from build123d import *

# Parameters (mm, degrees)
F1_DEPTH = 30
F2_R     = 2
F3_R     = 2
F4_R     = 25
F5_DEPTH = 30
F6_W     = 50
F6_H     = 19.9247
F7_DEPTH = 60


with BuildPart() as f1:
    # F0 (on Front) → F1 (new body, symmetric)
    with BuildSketch(Plane.XZ):
        with BuildLine():
            Line((27.891926, 68.585901), (-22.108074, 68.585901))
            ThreePointArc((-22.108074, 68.585901), (-39.785743, 61.263571), (-47.108074, 43.585901))
            Line((-47.108074, 43.585901), (-47.108074, -6.414099))
            ThreePointArc((-47.108074, -6.414099), (-39.785743, -24.091768), (-22.108074, -31.414099))
            Line((-22.108074, -31.414099), (27.891926, -31.414099))
            ThreePointArc((27.891926, -31.414099), (45.569596, -24.091768), (52.891926, -6.414099))
            Line((52.891926, -6.414099), (52.891926, 43.585901))
            ThreePointArc((52.891926, 43.585901), (45.569596, 61.263571), (27.891926, 68.585901))
        make_face()
    extrude(amount=F1_DEPTH, both=True)

    # F2
    f2_edges = [f1.edges().sort_by_distance(p)[0] for p in [
        (52.891926, 30, 18.585901),
        (45.569596, 30, 61.263571),
        (2.891926, 30, 68.585901),
        (-39.785743, 30, 61.263571),
        (-47.108074, 30, 18.585901),
        (-39.785743, 30, -24.091768),
        (2.891926, 30, -31.414099),
        (45.569596, 30, -24.091768),
    ]]
    fillet(f2_edges, radius=F2_R)

    # F3
    f3_edges = [f1.edges().sort_by_distance(p)[0] for p in [
        (52.891926, -30, 18.585901),
        (45.569596, -30, 61.263571),
        (2.891926, -30, 68.585901),
        (-39.785743, -30, 61.263571),
        (-47.108074, -30, 18.585901),
        (-39.785743, -30, -24.091768),
        (2.891926, -30, -31.414099),
        (45.569596, -30, -24.091768),
    ]]
    fillet(f3_edges, radius=F3_R)

    # F4 (on face) → F5 (cut)
    with BuildSketch(Plane.XZ.offset(30)):
        with Locations((3.43938, 20.517696)):
            Circle(F4_R)
    extrude(amount=-F5_DEPTH, mode=Mode.SUBTRACT)

    # F6 (on face) → F7 (cut)
    with BuildSketch(Plane.XY.offset(68.585901)):
        with Locations((2.891926, 0.830196)):
            Rectangle(F6_W, F6_H)
    extrude(amount=-F7_DEPTH, mode=Mode.SUBTRACT)


solid = f1.part
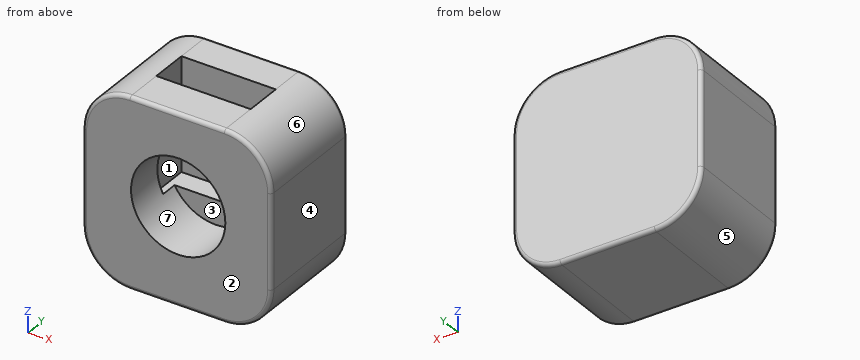
Read the model definition and answer for the solid it produces. Units are mm, in the model's axes. Face numbers are marked on the shaded views. A direction names the side the tool comes from. Round coordinates to 2 decimals unless told otherwise and drop trailing zeros. Order: outer loops, then holes, each group sorted by start corner. A loop starts at its lowest first (then second) coordinate and runs counter-clockwise, first axis right, second up.
1) The part is cut by section B-B on z = 23. Write down the section's boundary in (x, y), plus the area to 3 significant figures.
2) The part is cut by section C-C on x = -7. Write down the section's boundary in (y, z).
3) The part is cut by section D-D on y = 9. Write down the section's boundary in (x, z).
4) The mould has two halves that part along Z. Classify the marked faces 4, 5, 6 and 7: released by +Z, released by -Z, zero draft, split by the parting line, or undercut.
5) For the marked faces 1, 2 and 3, determine the directions among +Z, -Z, +X, -X, +Y, -Y from which every point of the face is accessible in a straight line to the end or side of a thin tool.
6) Straight lines are drawn through the part: L1, parallel to Y at x = 22, z = 61.5; L2, parallel to X at y = -20.5, z = 21.5; L3, parallel to X at y = 6.5, z = 17. For each, find the intervals that lie inside material, in ascending order.
7) Flat-ended cylindrical pins translate along their axes: pin 1 (14.5 mm diameter, centred on x = 12, z = 2, fed in from -Y); pin 2 (1 mm diameter, centred on x = 42, y = -10, fed in from +Z); pin 3 (3 mm diameter, centred on x = 13, z = 40.5, fed in from -Y); pin 4 (16 mm diameter, centred on x = -5.5, y = -0.5, fed in from +Z). Find the tip coordinate at first contact, or state that the pin passes through.
8) The part is cut by section A-A on y = 18. Write down the section's boundary in (x, z), plus the area to 3 significant figures.
Resolved:
1. outline: (-47.11, -28) arc R2 ccw to (-45.11, -30) - (-21.44, -30) - (-21.44, -9.13) - (-22.11, -9.13) - (-22.11, 10.79) - (27.89, 10.79) - (27.89, 0) - (28.32, 0) - (28.32, -30) - (50.89, -30) arc R2 ccw to (52.89, -28) - (52.89, 28) arc R2 ccw to (50.89, 30) - (-45.11, 30) arc R2 ccw to (-47.11, 28) - close
1. area: 3,960 mm2
2. outline: (-30, -29.41) arc R2 ccw to (-28, -31.41) - (28, -31.41) arc R2 ccw to (30, -29.41) - (30, 66.59) arc R2 ccw to (28, 68.59) - (10.79, 68.59) - (10.79, 8.59) - (0, 8.59) - (0, -2.2) - (-30, -2.2) - close; (-30, 43.23) - (-9.13, 43.23) - (-9.13, 68.59) - (-28, 68.59) arc R2 ccw to (-30, 66.59) - close
3. outline: (-47.11, -6.41) arc R25 ccw to (-22.11, -31.41) - (27.89, -31.41) arc R25 ccw to (52.89, -6.41) - (52.89, 43.59) arc R25 ccw to (27.89, 68.59) - (27.89, 8.59) - (-22.11, 8.59) - (-22.11, 68.59) arc R25 ccw to (-47.11, 43.59) - close
4. face 4: zero draft
4. face 5: released by -Z
4. face 6: released by +Z
4. face 7: undercut
5. face 1: +Z
5. face 2: +Z, -Z, +X, -X, -Y
5. face 3: +Z, -Y
6. L1: y = -30 to -9.13, 10.79 to 30
6. L2: x = -47.11 to -21.54, 28.42 to 52.89
6. L3: x = -47.11 to -22.11, 27.89 to 52.89
7. pin 1: stops at y = -30
7. pin 2: stops at z = 64.56
7. pin 3: stops at y = 10.79
7. pin 4: stops at z = 8.59
8. outline: (-47.11, -6.41) arc R25 ccw to (-22.11, -31.41) - (27.89, -31.41) arc R25 ccw to (52.89, -6.41) - (52.89, 43.59) arc R25 ccw to (27.89, 68.59) - (-22.11, 68.59) arc R25 ccw to (-47.11, 43.59) - close
8. area: 9,460 mm2
